Autodesk Inventor part; units mm, degrees
ref_plane "YZ Plane" through (0, 0, 0) normal (1, 0, 0) x (0, 1, 0)
ref_plane "XZ Plane" through (0, 0, 0) normal (0, 1, 0) x (-1, 0, 0)
ref_plane "XY Plane" through (0, 0, 0) normal (0, 0, 1) x (1, 0, 0)
sketch "スケッチ1" plane through (0, 0, 0) normal (0, 0, 1) x (1, 0, 0)
  circle A0 centre (0, 0) radius 3
  line L0 (0, 3) -> (0, -3) construction
  line L1 (-0.5, 2.958) -> (-0.5, -2.958)
  line L2 (0.5, 2.958) -> (0.5, -2.958)
  dimension "d0" = 6
  dimension "d1" = 1
extrude "押し出し1" add sketch "スケッチ1" along normal blind 13
extrude "押し出し2" cut sketch "スケッチ1" along normal blind 1 contours L2 A0 L1
chamfer "面取り1" distance 0.3 angle 45 4 edges at (-3, 0, 13) (2.2913, 1.9365, 0) (2.2913, -1.9365, 0) (-3, 0, 0)
hole "穴1" at (0, 0, 0) direction (0, 0, 1) diameter 2.459 end through all
properties part number "ARL-313SBE" material "アルミニウム 2014-T4"
Can you work these out from the model? Positions are in its coordinate system, mm. A direction names the side the tool comes from. Give positions to 0.01 mm unless a question says otherwise; leave off trailing zeros. Loops run counter-clockwise (first coordinate to the right, second up) from the corner with the lowest first, then second, coordinate; pieces in that order, holes last. Notation, with made-up numbers: (-6.75, 17.25) - (1.25, 17.25) arc R21 ccw to (1.25, 23.25) - close; hole circle Ø11 at (86, 86.5). An arc over 180 degrees is marked (long way). One line per item, written item: value.
(1) On a 3-axis mill with a long thin cutter (end or side, diameter ignored), from which of +Z, -Z, +X, -X, +Y, -Y can I reach the whole of each face in a straight line? I mean faces 1 (the face through (0, -2, 1)), 2 (the face through (-2.82, -0.05, 12.88)). Say none if no direction works.
Verdict:
face 1: -Z, +Y, -Y
face 2: +Z, -X
(2) If we section it at B-B, the plane y = 0: List the corners of the cut face in (x, z) for me.
Verdict:
outline: (-3, 0.3) - (-2.7, 0) - (-1.23, 0) - (-1.23, 13) - (-2.7, 13) - (-3, 12.7) - close; (1.23, 0) - (2.7, 0) - (3, 0.3) - (3, 12.7) - (2.7, 13) - (1.23, 13) - close
(3) If we section it at A-A, the plane x = 0: List the corners of the cut face in (y, z) for me, plus the area to 3 significant figures.
Verdict:
outline: (-3, 1) - (-1.23, 1) - (-1.23, 13) - (-2.7, 13) - (-3, 12.7) - close; (1.23, 1) - (3, 1) - (3, 12.7) - (2.7, 13) - (1.23, 13) - close
area: 42.4 mm^2
(4) I'm going to push flat-ended pins straight in: pin 1 (1.5 mm diameter, centred on y = 1.5, z = 11, fed in from -X); pin 2 (1.1 mm diameter, centred on y = 2.5, z = 0.5, fed in from -X); pin 3 (0.5 mm diameter, centred on x = 0, y = -2, fed in from -Z). Where does each tip first touch, or does it pass through?
Verdict:
pin 1: x = -2.9
pin 2: x = -2.28
pin 3: z = 1
(5) If we mould it in two halves opening along X, with no side actions, what happens to faces 3 (the face through (2, 0, 0)), 4 (the face through (-0.5, 2.1, 0.5)), 5 (the face through (2.82, 0.05, 12.88))? For each: released by +X, released by -X, zero draft, split by the parting line, or undercut.
Verdict:
face 3: zero draft
face 4: undercut
face 5: released by +X
(6) I need wall thicknesses on line 1 along Y through (x, z) = (0, 5.25); line 2 along X through (y, z) = (-0.5, 5). Which ranges of each line are inside material? Lowest first, please.
Verdict:
line 1: -3 to -1.23, 1.23 to 3
line 2: -2.96 to -1.12, 1.12 to 2.96
(7) If we section it at C-C, the plane z = 4.5: List the corners of the cut face in (x, y) for me, plus the area to 3 significant figures.
Verdict:
outline: circle Ø6 at (0, 0); hole circle Ø2.46 at (0, 0)
area: 23.5 mm^2
